from build123d import *

# Parameters (mm, degrees)
F0_W           = 50.8
F0_H           = 50.8
F1_DEPTH       = 76.2
F3_D           = 6.7564
F3_CSINK_D     = 25.4
F3_CSINK_ANGLE = 82


with BuildPart() as f1:
    # F0 (on Front) → F1 (new body)
    with BuildSketch(Plane.XZ):
        with Locations((25.4, 25.4)):
            Rectangle(F0_W, F0_H)
    extrude(amount=F1_DEPTH)

    # F3 (through all)
    with Locations(Plane.XY.offset(50.8)):
        with Locations((25.4, -38.1)):
            CounterSinkHole(F3_D / 2, F3_CSINK_D / 2, counter_sink_angle=F3_CSINK_ANGLE)


solid = f1.part
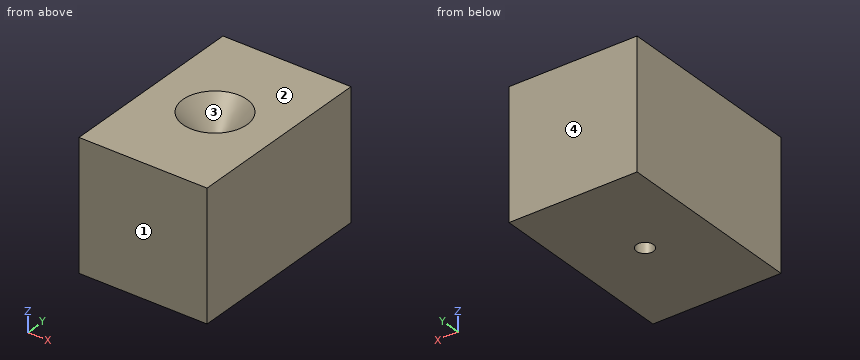
Source: CAD feature listing. Evaluate the final solid. Frame: model axes, mm. Face numbers are marked on the shaded views. Round coordinates to 2 decimals unless told otherwise and drop trailing zeros. Loops run counter-clockwise (first coordinate to the right, second up) from the corner with the lowest first, then second, coordinate; pieces in that order, holes last. Notation, with made-up numbers: (-34, -23.5) - (-8, -23.5) arc R32 cw to (-8, 12.5) - close; hole circle Ø9 at (-2, -32.75). An arc over 180 degrees is marked (long way). Write item = value, one per line. Start each with the question number.
Item 1: First-contact query: pin 1 Ø1.5 at (x, z) = (28.5, 16) entering from +Y; pin 2 Ø6 at (x, y) = (25.4, -38.1) entering from +Z. Flat tips, straight axial feed; report the tip coordinate or a pass-through.
Item 2: Section query A-A on x = 25.4. Output: boundary loops of the cut face in (y, z).
Item 3: Mould query, pull axis Y, two halves, no side actions, for the marked faces 1, 2, 3 and 4. Classes: released by +Y, released by -Y, zero draft, split by the parting line, or undercut.
Item 4: Section query B-B on y = -38.1. Output: boundary loops of the cut face in (x, z), plus the area to 3 significant figures.
Item 5: Material intervals for line 1 (X direction, y = -38, z = 26); line 2 (Y direction, x = 25.4, z = 11); line 3 (Y direction, x = 26.5, z = 40), sorted ascending.
Results list:
q1.pin_1 = 0
q1.pin_2 = through
q2.outline = (-76.2, 0) - (-41.48, 0) - (-41.48, 40.08) - (-50.8, 50.8) - (-76.2, 50.8) - close; (-34.72, 0) - (0, 0) - (0, 50.8) - (-25.4, 50.8) - (-34.72, 40.08) - close
q3.face_1 = released by -Y
q3.face_2 = zero draft
q3.face_3 = undercut
q3.face_4 = released by +Y
q4.outline = (0, 0) - (22.02, 0) - (22.02, 40.08) - (12.7, 50.8) - (0, 50.8) - close; (28.78, 0) - (50.8, 0) - (50.8, 50.8) - (38.1, 50.8) - (28.78, 40.08) - close
q4.area = 2,140 mm²
q5.line_1 = 0 to 22.02, 28.78 to 50.8
q5.line_2 = -76.2 to -41.48, -34.72 to 0
q5.line_3 = -76.2 to -41.29, -34.91 to 0
